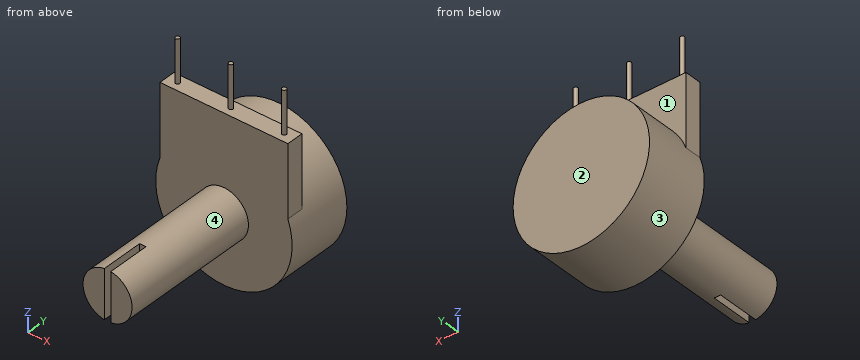
from build123d import *

# Parameters (mm, degrees)
F0_R     = 8.128
F1_DEPTH = 7.9248
F2_R     = 2.921
F3_DEPTH = 16.8402
F4_W     = 15.24
F4_H     = 10.8462307572
F5_DEPTH = 2.032
F6_R     = 0.254
F7_DEPTH = 5.08
F8_W     = 0.762
F8_H     = 6.35
F9_DEPTH = 5.08


with BuildPart() as f1:
    # F0 (on Front) → F1 (new body)
    with BuildSketch(Plane.XZ):
        Circle(F0_R)
    extrude(amount=F1_DEPTH)

    # F2 (on face) → F3 (join)
    with BuildSketch(Plane.XZ.offset(7.9248)):
        Circle(F2_R)
    extrude(amount=F3_DEPTH)

    # F4 (on face) → F5 (join)
    with BuildSketch(Plane.XZ.offset(7.9248)):
        with Locations((0, 5.9306846214)):
            Rectangle(F4_W, F4_H)
    extrude(amount=-F5_DEPTH)

    # F6 (on face) → F7 (join)
    with BuildSketch(Plane.XY.offset(11.3538)):
        with Locations((0, -6.9088)):
            Circle(F6_R)
        with Locations((6.35, -6.9088)):
            Circle(F6_R)
        with Locations((-6.35, -6.9088)):
            Circle(F6_R)
    extrude(amount=F7_DEPTH)

    # F8 (on face) → F9 (cut)
    with BuildSketch(Plane.XZ.offset(24.765)):
        Rectangle(F8_W, F8_H)
    extrude(amount=-F9_DEPTH, mode=Mode.SUBTRACT)


solid = f1.part
Could you check a few things on this model? Use its own coordinates, in mm. Face numbers are marked on the shaded views. A direction names the side the tool comes from. Round coordinates to 2 decimals unless told otherwise and drop trailing zeros. Order: outer loops, then holes, each group sorted by start corner. A loop starts at its lowest first (then second) coordinate and runs counter-clockwise, first axis right, second up.
Q1. Imagine slicing it at D-D, the plane z = 10. List the corners of the cut face in (x, y) for me, then the cut area to 3 significant figures.
Geometry says:
outline: (-7.62, -7.92) - (7.62, -7.92) - (7.62, -5.89) - (-7.62, -5.89) - close
area: 31.0 mm2
Q2. I'm going to push flat-ended pins straight in: P1, Ø2, axis at x = 1.5, y = -7, coming from the +Z side; P2, Ø1, axis at y = -6.5, z = 8, coming from the +X side; P3, Ø8, axis at x = 3, z = 2.5, coming from the -Y side (3 decimals); P4, Ø2, axis at x = 4, z = 9.5, coming from the +Y side. Where does each tip first touch, or does it pass through?
Geometry says:
P1: stops at z = 11.35
P2: stops at x = 7.62
P3: stops at y = -24.765
P4: stops at y = -5.89
Q3. Which directions (+Z, -Z, +X, -X, +Y, -Y) give clear straight access to the entire face, cutting with the end or side of a thin tool? Please do the marked faces 1, 2, 3 and 4.
Geometry says:
face 1: +Z, +Y
face 2: +Z, -Z, +X, -X, +Y
face 3: +Y
face 4: -Y
Q4. Imagine slicing it at A-A, the plane z = 0. List the corners of the cut face in (x, y) for me (3 decimals).
Geometry says:
outline: (-8.128, -7.925) - (-2.921, -7.925) - (-2.921, -24.765) - (-0.381, -24.765) - (-0.381, -19.685) - (0.381, -19.685) - (0.381, -24.765) - (2.921, -24.765) - (2.921, -7.925) - (8.128, -7.925) - (8.128, 0) - (-8.128, 0) - close
Q5. Please list where these lines run through material, in increasing order: probe 1 along Y at (x, z) = (3.5, 3.25); probe 2 along Y at (x, z) = (-0.25, 0.5) (3 decimals); probe 3 along X at (y, z) = (-4.25, 4.75).
Geometry says:
probe 1: y = -7.92 to 0
probe 2: y = -19.685 to 0
probe 3: x = -6.6 to 6.6
Q6. Imagine slicing it at C-C, the plane y = -4. List the corners of the cut face in (x, z) for me, then the cut area to 3 significant figures.
Geometry says:
outline: circle Ø16.26 at (0, 0)
area: 208 mm2
